Here's how the part is built. I have some questions about the finished solid (model axes, mm). Coordinates: 2 decimals unless noted, no trailing zeros. Loops run counter-clockwise (first coordinate to the right, second up) from the corner with the lowest first, then second, coordinate; pieces in that order, holes last. Notation, with made-up numbers: (-2.5, 12.5) -> (54.5, 12.5) arc R29 ccw to (54.5, 37.5) -> close; hole circle Ø3 at (-35, -26.5). An arc over 180 degrees is marked (long way). Answer as a JSON object with one key per item and string values. Group by question number.
Q1. Thinking about a two-plate mould opening in X: for faces 1 (the flat face through (-4, 0, -15)), 2 (the cylindrical face through (-71.646, 2.028, -9.355)), 3 (the cylindrical face through (67.483, 2.028, -25.26)), 4 (the flat face through (112.5, 2, -11)), which applies, released by +X, released by -X, zero draft, split by the parting line, or undercut?
Q2. I'm going to push a flat-ended pin straight in: pin 1 (3 mm diameter, centred on x = 102.5, z = -15, fed in from +Y). Where does the tip first touch, or does it pass through?
Q3. I want a section at B-B on x = 79. Write out the boundary of the cut face in (y, z).
Q4. I need wall thicknesses on line 1 (X direction, y = 1.9, z = -15); line 2 (X direction, y = 0.2, z = -7.5); line 3 (X direction, y = 1.4, z = -16.8). Which ranges of each line are inside material? Lowest first, please.
Q5. I want a section at A-A on y = 2.45. Count the separate pieces of the cut face and the enclosed holes in it, then the cut area to 3 significant figures.
```python
from build123d import *

# Parameters (mm, degrees)
SKETCH1_W           = 225
SKETCH1_H           = 38
BOSS_EXTRUDE1_DEPTH = 4
CUT_EXTRUDE1_REACH  = 118.5
SKETCH2_R           = 10.5
SKETCH2_R_2         = 5.5
SKETCH10_W          = 5
SKETCH10_H          = 38
BOSS_EXTRUDE2_DEPTH = 4
SKETCH11_R          = 2
CUT_EXTRUDE2_DEPTH  = 27
SKETCH12_R          = 2
CUT_EXTRUDE3_DEPTH  = 27
SKETCH14_R          = 1.5
CUT_EXTRUDE4_DEPTH  = 10
CIRPATTERN1_COUNT   = 4


with BuildPart() as part:
    # Sketch1 → Boss-Extrude1 (new body)
    with BuildSketch(Plane(origin=(0, 0, 0), x_dir=(1, 0, 0), z_dir=(0, 1, 0))):
        with Locations((0, 11)):
            Rectangle(SKETCH1_W, SKETCH1_H)
    extrude(amount=BOSS_EXTRUDE1_DEPTH)

    # Sketch2 → Cut-Extrude1 (cut, up to next)
    with BuildSketch(Plane(origin=(0, 4, 0), x_dir=(1, 0, 0), z_dir=(0, 1, 0)), mode=Mode.PRIVATE) as cut_extrude1_sk1:
        with Locations(Location((75.5, 15, 0), (0, 0, 270))):
            Circle(SKETCH2_R)
    cut_extrude1_tool1 = extrude(cut_extrude1_sk1.sketch, amount=-CUT_EXTRUDE1_REACH, mode=Mode.PRIVATE) & part.part
    # Sketch2 → Cut-Extrude1 (cut, up to next)
    with BuildSketch(Plane(origin=(0, 4, 0), x_dir=(1, 0, 0), z_dir=(0, 1, 0)), mode=Mode.PRIVATE) as cut_extrude1_sk2:
        with Locations(Location((-80.5, 15, 0), (0, 0, 270))):
            Circle(SKETCH2_R)
    cut_extrude1_tool2 = extrude(cut_extrude1_sk2.sketch, amount=-CUT_EXTRUDE1_REACH, mode=Mode.PRIVATE) & part.part
    # Sketch2 → Cut-Extrude1 (cut, up to next)
    with BuildSketch(Plane(origin=(0, 4, 0), x_dir=(1, 0, 0), z_dir=(0, 1, 0)), mode=Mode.PRIVATE) as cut_extrude1_sk3:
        with Locations(Location((-2.5, 8.7, 0), (0, 0, 270))):
            Circle(SKETCH2_R_2)
    cut_extrude1_tool3 = extrude(cut_extrude1_sk3.sketch, amount=-CUT_EXTRUDE1_REACH, mode=Mode.PRIVATE) & part.part
    add(cut_extrude1_tool1.solids().sort_by_distance((75.5, 4, -15))[0], mode=Mode.SUBTRACT)
    add(cut_extrude1_tool2.solids().sort_by_distance((-80.5, 4, -15))[0], mode=Mode.SUBTRACT)
    add(cut_extrude1_tool3.solids().sort_by_distance((-2.5, 4, -8.7))[0], mode=Mode.SUBTRACT)

    # Sketch10 → Boss-Extrude2 (add)
    with BuildSketch(Plane(origin=(0, 4, 0), x_dir=(1, 0, 0), z_dir=(0, 1, 0))):
        with Locations((-115, 11)):
            Rectangle(SKETCH10_W, SKETCH10_H)
        with Locations((100, 11)):
            Rectangle(SKETCH10_W, SKETCH10_H)
    extrude(amount=-BOSS_EXTRUDE2_DEPTH)

    # Sketch11 → Cut-Extrude2 (cut)
    with BuildSketch(Plane(origin=(0, 4, 0), x_dir=(1, 0, 0), z_dir=(0, 1, 0))):
        with Locations(Location((102.5, 0, 0), (0, 0, 270))):
            Circle(SKETCH11_R)
        with Locations(Location((102.5, 15, 0), (0, 0, 270))):
            Circle(SKETCH11_R)
        with Locations(Location((-107.5, 15, 0), (0, 0, 270))):
            Circle(SKETCH11_R)
        with Locations(Location((-107.5, 0, 0), (0, 0, 270))):
            Circle(SKETCH11_R)
    extrude(amount=-CUT_EXTRUDE2_DEPTH, mode=Mode.SUBTRACT)

    # Sketch12 → Cut-Extrude3 (cut)
    with BuildSketch(Plane(origin=(0, 4, 0), x_dir=(1, 0, 0), z_dir=(0, 1, 0))):
        with Locations(Location((65.5, 5, 0), (0, 0, 270))):
            Circle(SKETCH12_R)
        with Locations(Location((85.5, 5, 0), (0, 0, 270))):
            Circle(SKETCH12_R)
        with Locations(Location((85.5, 25, 0), (0, 0, 270))):
            Circle(SKETCH12_R)
        with Locations(Location((65.5, 25, 0), (0, 0, 270))):
            Circle(SKETCH12_R)
        with Locations(Location((-70.5, 25, 0), (0, 0, 270))):
            Circle(SKETCH12_R)
        with Locations(Location((-90.5, 25, 0), (0, 0, 270))):
            Circle(SKETCH12_R)
        with Locations(Location((-90.5, 5, 0), (0, 0, 270))):
            Circle(SKETCH12_R)
        with Locations(Location((-70.5, 5, 0), (0, 0, 270))):
            Circle(SKETCH12_R)
    extrude(amount=-CUT_EXTRUDE3_DEPTH, mode=Mode.SUBTRACT)

    # Sketch14 → Cut-Extrude4 (cut)
    with BuildSketch(Plane(origin=(0, 4, 0), x_dir=(1, 0, 0), z_dir=(0, 1, 0))):
        with Locations(Location((-2.5, 16.8, 0), (0, 0, 270))):
            Circle(SKETCH14_R)
    cut_extrude4 = extrude(amount=-CUT_EXTRUDE4_DEPTH, mode=Mode.SUBTRACT)

    # CirPattern1: Cut-Extrude4 ×4 about axis
    cirpattern1_axis = Axis((-2.5, 0, -8.7), (0, 1, 0))
    for i in range(1, CIRPATTERN1_COUNT):
        add(cut_extrude4.rotate(cirpattern1_axis, i * 360 / CIRPATTERN1_COUNT), mode=Mode.SUBTRACT)


solid = part.part
```
Result set:
{
 "1": {"face 1": "zero draft", "face 2": "undercut", "face 3": "undercut", "face 4": "released by +X"},
 "2": {"pin 1": "passes through"},
 "3": {"outline": "(0, -30) -> (4, -30) -> (4, -24.9) -> (0, -24.9) -> close; (0, -5.1) -> (4, -5.1) -> (4, 8) -> (0, 8) -> close"},
 "4": {"line 1": "x = -117.5 to -109.5, -105.5 to -91, -70 to 65, 86 to 100.5, 104.5 to 112.5", "line 2": "x = -117.5 to -87.85, -73.15 to -11.5, -9.7 to -7.87, 2.87 to 4.7, 6.5 to 68.15, 82.85 to 112.5", "line 3": "x = -117.5 to -108.37, -106.63 to -90.84, -70.16 to -4, -1 to 65.16, 85.84 to 101.63, 103.37 to 112.5"},
 "5": {"separate pieces": "1", "enclosed holes": "19", "area": "7,770 mm²"}
}
